from build123d import *

# Parameters (mm, degrees)
BOSS_EXTRUDE1_DEPTH = 3.175


with BuildPart() as part:
    # Sketch1 → Boss-Extrude1 (new body)
    with BuildSketch(Plane(origin=(0, 0, 0), x_dir=(0, 0, -1), z_dir=(1, 0, 0))):
        Polygon((-7.9375, 0), (-7.9375, -162.306), (4.7625, -162.306), (4.7625, -155.956), (4.7625, -143.256), (4.7625, -127.3048), (4.7625, -114.6048), (7.9375, -114.6048), (7.9375, -98.6536), (4.7625, -98.6536), (4.7625, -85.9536), (7.9375, -85.9536), (7.9375, -70.0024), (4.7625, -70.0024), (4.7625, -57.3024), (7.9375, -57.3024), (7.9375, -41.3512), (4.7625, -41.3512), (4.7625, -28.6512), (7.9375, -28.6512), (7.9375, -12.7), (4.7625, -12.7), (4.7625, 0), align=None)
    extrude(amount=BOSS_EXTRUDE1_DEPTH)


solid = part.part
CAD build for the part. Positions are in the model's coordinates, mm. A direction names the side the tool comes from. Give positions to 0.01 mm unless a question says otherwise; leave off trailing zeros. Loops run counter-clockwise (first coordinate to the right, second up) from the corner with the lowest first, then second, coordinate; pieces in that order, holes last. Notation, with made-up numbers: M 50,63 L 61,63 A32 cw 61,100 Z; hole C -39.5,4 d1. An arc over 180 degrees is marked long. Answer in a Markdown table with one row per item. Add a question column.
Item 1: Mould opens along Y. For faces 5 (the face through (0, -80, 2)), 6 (the face through (2, -85.954, -6)), 7 (the face through (2, -162.306, 2)), 8 (the face through (2, 0, 1)) say: +Y half, -Y half, draft (parallel to the pull), parting line (faces both ways), or undercut.
Item 2: Probe probe 1 along Y at (x, z) = (2.95, -6); probe 2 along Z at (x, y) = (2.15, -66.5). List the from-to ranges inside material, lowest first.
Item 3: Band-saw the part on A-A on x = 2.1. Give the cut face in (y, z), then the cut area to 3 significant figures.
Item 4: Tool access for faces 1 (the face through (2, -6, -4.762)), 2 (the face through (2, -139, -4.762)), 3 (the face through (2, -70.002, -6)), 4 (the face through (2, -80, 7.938)): list every direction of +Z, -Z, +X, -X, +Y, -Y with a clear straight run to the whole face (end or side of a thin tool).
Item 5: Drop flat-ended pins along their axis: P1, Ø1, axis at x = 1.5, y = -8, coming from the -Z side; P2, Ø1, axis at x = 1.5, z = -7, coming from the +Y side; P3, Ø1, axis at x = 1, z = -7, coming from the -Y side. Give the stop position or say it passes through.
Item 6: Band-saw the part on B-B on y = -134.5. Give the cut face in (x, z) (1 decimal).
Reply:
| question | item | result |
|---|---|---|
| 1 | face 5 | draft |
| 1 | face 6 | undercut |
| 1 | face 7 | -Y half |
| 1 | face 8 | +Y half |
| 2 | probe 1 | y = -114.6 to -98.65, -85.95 to -70, -57.3 to -41.35, -28.65 to -12.7 |
| 2 | probe 2 | z = -4.76 to 7.94 |
| 3 | outline | M -162.31,-4.76 L -114.6,-4.76 L -114.6,-7.94 L -98.65,-7.94 L -98.65,-4.76 L -85.95,-4.76 L -85.95,-7.94 L -70,-7.94 L -70,-4.76 L -57.3,-4.76 L -57.3,-7.94 L -41.35,-7.94 L -41.35,-4.76 L -28.65,-4.76 L -28.65,-7.94 L -12.7,-7.94 L -12.7,-4.76 L 0,-4.76 L 0,7.94 L -162.31,7.94 Z |
| 3 | area | 2,260 mm^2 |
| 4 | face 1 | -Z, +X, -X, +Y |
| 4 | face 2 | -Z, +X, -X, -Y |
| 4 | face 3 | -Z, +X, -X |
| 4 | face 4 | +Z, +X, -X, +Y, -Y |
| 5 | P1 | stops at z = -4.76 |
| 5 | P2 | stops at y = -12.7 |
| 5 | P3 | stops at y = -114.6 |
| 6 | outline | M 0,-4.8 L 3.2,-4.8 L 3.2,7.9 L 0,7.9 Z |
